Design review of the part built by this model. Coordinates are the model's own, in mm. Face numbers are marked on the shaded views. A direction names the side the tool comes from. Give positions to 0.01 mm unless a question says otherwise; leave off trailing zeros. Loops run counter-clockwise (first coordinate to the right, second up) from the corner with the lowest first, then second, coordinate; pieces in that order, holes last. Notation, with made-up numbers: (36, 1) -> (93, 1) arc R7 ccw to (93, 10) -> close; hole circle Ø4 at (79, 80.5). An arc over 180 degrees is marked (long way). Use a Markdown table: item, result. Add a question column.
1. Draft analysis for pull direction Z (two halves, no side actions). For the marked faces 1, 2, 3 and 4, state which applies: pulls with the +Z half, pulls with the -Z half, needs draft (parallel to the pull), parting line crosses it, or undercut.
2. For the marked faces 5 and 6, list the 3-axis set-ups (+Z, -Z, +X, -X, +Y, -Y) from which the entire face can be reached by the end or side of a thin tool; tool diameter is ignored.
3. Add section B-B (z = 0). State the section outline as (x, y) points.
4. Add section C-C (y = 6.5). State the section outline as (x, z) points, and give its area (3 significant figures).
5. To check wall thickness, follow line 1 (X direction, y = 7.85, z = -18.5); line 2 (Z direction, x = -18.5, y = 8.4); line 3 (Z direction, x = -18.5, y = 6.15). State the ranges of each line that lie inside material, in increasing order.
6. Add section A-A (x = 18.5). State the section outline as (y, z) points, and give its area (3 significant figures).
7. Add section D-D (x = -7). State the section outline as (y, z) points.
8. For pin 1 Ø3.5 at (x, z) = (18, 19) entering from +Y; pin 2 Ø2.5 at (y, z) = (5.5, -0.5) entering from +X, all flat-tipped, find the tip position at first contact; note any pin that passes through.
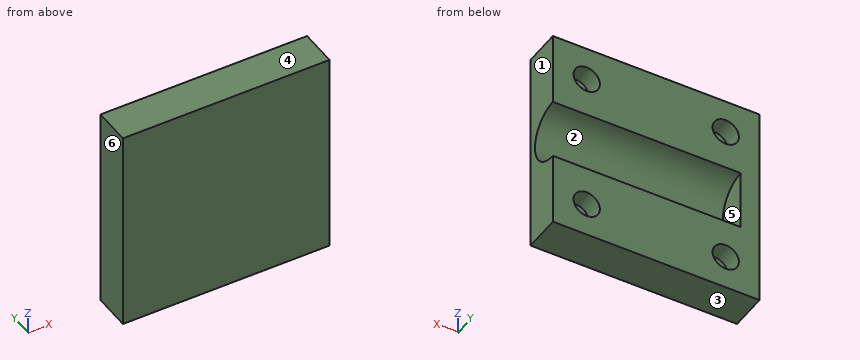
```python
from build123d import *

# Parameters (mm, degrees)
SKETCH1_W           = 55
SKETCH1_H           = 55
BOSS_EXTRUDE1_DEPTH = 10
SKETCH2_R           = 8
CUT_EXTRUDE1_DEPTH  = 50
SKETCH3_R           = 3.5
CUT_EXTRUDE2_DEPTH  = 5


with BuildPart() as part:
    # Sketch1 → Boss-Extrude1 (new body)
    with BuildSketch(Plane(origin=(0, 0, 0), x_dir=(1, 0, 0), z_dir=(0, 1, 0))):
        Rectangle(SKETCH1_W, SKETCH1_H)
    extrude(amount=BOSS_EXTRUDE1_DEPTH)

    # Sketch2 → Cut-Extrude1 (cut)
    with BuildSketch(Plane(origin=(27.5, 0, 0), x_dir=(0, 0, -1), z_dir=(1, 0, 0))):
        with Locations((0, 10)):
            Circle(SKETCH2_R)
    extrude(amount=-CUT_EXTRUDE1_DEPTH, mode=Mode.SUBTRACT)

    # Sketch3 → Cut-Extrude2 (cut)
    with BuildSketch(Plane(origin=(0, 10, 0), x_dir=(1, 0, 0), z_dir=(0, 1, 0))):
        with Locations((-18.5, 18.5)):
            Circle(SKETCH3_R)
        with Locations((18.5, 18.5)):
            Circle(SKETCH3_R)
        with Locations((-18.5, -18.5)):
            Circle(SKETCH3_R)
        with Locations((18.5, -18.5)):
            Circle(SKETCH3_R)
    extrude(amount=-CUT_EXTRUDE2_DEPTH, mode=Mode.SUBTRACT)


solid = part.part
```
Taken from the geometry:
| question | item | result |
|---|---|---|
| 1 | face 1 | needs draft |
| 1 | face 2 | undercut |
| 1 | face 3 | pulls with the -Z half |
| 1 | face 4 | pulls with the +Z half |
| 2 | face 5 | +X, +Y |
| 2 | face 6 | +Z, -Z, -X, +Y, -Y |
| 3 | outline | (-27.5, 0) -> (27.5, 0) -> (27.5, 2) -> (-22.5, 2) -> (-22.5, 10) -> (-27.5, 10) -> close |
| 4 | outline | (-27.5, -27.5) -> (27.5, -27.5) -> (27.5, -7.19) -> (-22.5, -7.19) -> (-22.5, 7.19) -> (27.5, 7.19) -> (27.5, 27.5) -> (-27.5, 27.5) -> close; hole circle Ø7 at (-18.5, -18.5); hole circle Ø7 at (-18.5, 18.5); hole circle Ø7 at (18.5, -18.5); hole circle Ø7 at (18.5, 18.5) |
| 4 | area | 2,150 mm^2 |
| 5 | line 1 | x = -27.5 to -22, -15 to 15, 22 to 27.5 |
| 5 | line 2 | z = -27.5 to -22, -15 to -7.84, 7.84 to 15, 22 to 27.5 |
| 5 | line 3 | z = -27.5 to -22, -15 to -7.01, 7.01 to 15, 22 to 27.5 |
| 6 | outline | (0, -27.5) -> (10, -27.5) -> (10, -22) -> (5, -22) -> (5, -15) -> (10, -15) -> (10, -8) arc R8 cw to (10, 8) -> (10, 15) -> (5, 15) -> (5, 22) -> (10, 22) -> (10, 27.5) -> (0, 27.5) -> close |
| 6 | area | 379 mm^2 |
| 7 | outline | (0, -27.5) -> (10, -27.5) -> (10, -8) arc R8 cw to (10, 8) -> (10, 27.5) -> (0, 27.5) -> close |
| 8 | pin 1 | stops at y = 5 |
| 8 | pin 2 | stops at x = -22.5 |
